Can you work these out from the drawing? Everything is in mm from the part's minimum corner. Round coordinates to 2 decimals unless told otherwise and drop trailing zeros. Write each loop counter-clockwise with the first axis right and the second up, starting at its lowest first coordinate (ties: lowest second). Pieces come first, ordered by that corner, then holes. Notation, with made-up numbers: (29.5, 53.5) -> (41.5, 53.5) arc R13 cw to (41.5, 73.5) -> close; hole circle Ø9 at (0.5, 7.25). An arc over 180 degrees is marked (long way). Answer as CSV lines item,"result".
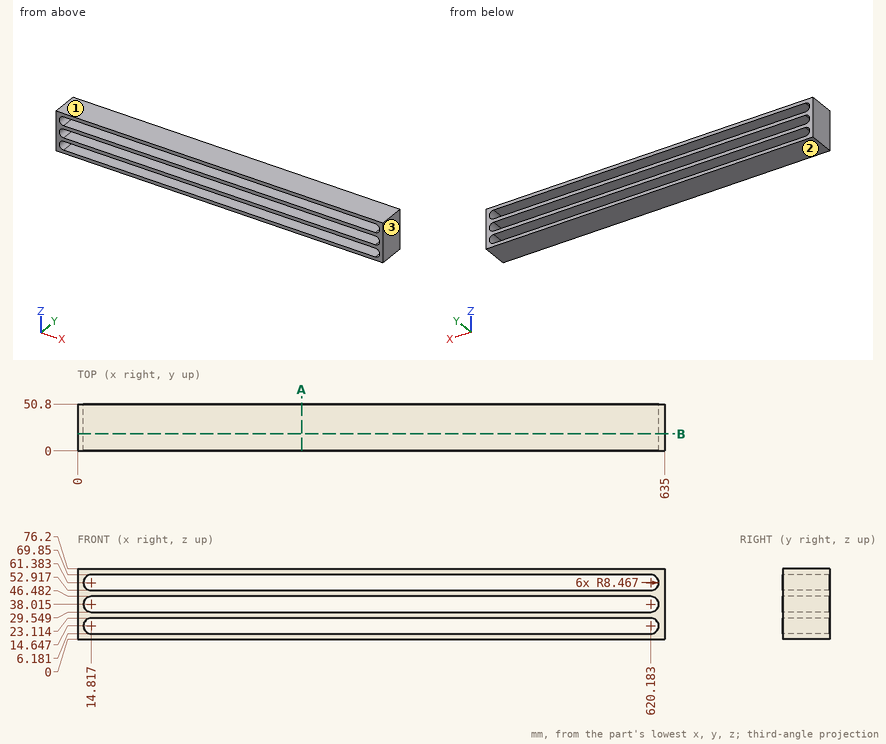
Item 1: Suppose I cut it at B-B, the plane y = 18.5. State how many separate pieces and enclosed holes the cut face has, then the cut area to 3 significant figures.
Results found:
separate pieces,"1"
enclosed holes,"3"
area,"17,000 mm²"
Item 2: Will this pin go through, and if not, where does the flat tip stop? pin 1 (8 mm diameter, centred on x = 165, z = 42, fed in from +Y).
Results found:
pin 1,"passes through"
Item 3: Suppose I cut it at A-A, the plane x = 242.5. List the corners of the cut face in (y, z) for me, then the cut area to 3 significant figures.
Results found:
outline,"(0, 0) -> (50.8, 0) -> (50.8, 6.18) -> (0, 6.18) -> close; (0, 23.11) -> (50.8, 23.11) -> (50.8, 29.55) -> (0, 29.55) -> close; (0, 46.48) -> (50.8, 46.48) -> (50.8, 52.92) -> (0, 52.92) -> close; (0, 69.85) -> (50.8, 69.85) -> (50.8, 76.2) -> (0, 76.2) -> close"
area,"1,290 mm²"
Item 4: I need wall thicknesses on L1, parallel to Z at x = 370, y = 20.5; L2, parallel to X at y = 15.5, z = 40 (1 decimal); L3, parallel to X at y = 11.5, z = 44.5 (1 decimal). Which ranges of each line are inside material? Lowest first, please.
Results found:
L1,"z = 0 to 6.18, 23.11 to 29.55, 46.48 to 52.92, 69.85 to 76.2"
L2,"x = 0 to 6.6, 628.4 to 635"
L3,"x = 0 to 9.4, 625.6 to 635"
Item 5: If we mould it in two halves opening along Z, with no side actions, what happens to the marked faces 1, 2 and 3? For each: pulls with the +Z half, pulls with the -Z half, needs draft (parallel to the pull), parting line crosses it, or undercut.
Results found:
face 1,"pulls with the +Z half"
face 2,"pulls with the -Z half"
face 3,"needs draft"
